```python
from build123d import *

# Parameters (mm, degrees)
F1_DEPTH = 1.5875


# Not quite as in the source:
# - a length typed as a fraction of an inch, garbled in the dataset ("3 / 203.2 mm" for 3/8 in), is restored


with BuildPart() as f1:
    # F0 (on Front) → F1 (new body)
    with BuildSketch(Plane.XZ):
        with BuildLine():
            ThreePointArc((-0.162727133, 0.4717287226), (0.0926759109, 0.1300044324), (0.4990071217, 0))
            Line((0.4990071217, 0), (22.65, 0))
            ThreePointArc((22.65, 0), (23.1449747468, 0.2050252532), (23.35, 0.7))
            Line((23.35, 0.7), (23.35, 7.5980762114))
            Line((23.35, 7.5980762114), (23.35, 8))
            Line((23.35, 8), (-12.65, 17.6461709275))
            Line((-12.65, 17.6461709275), (-12.65, 16.1461709275))
            ThreePointArc((-12.65, 16.1461709275), (-12.2964466094, 15.9997243181), (-12.15, 15.6461709275))
            ThreePointArc((-12.15, 15.6461709275), (-12.2964466094, 15.2926175369), (-12.65, 15.1461709275))
            Line((-12.65, 15.1461709275), (-12.65, 7.6820693124))
            Line((-12.65, 7.6820693124), (-6.2143365838, 7.6820693124))
            ThreePointArc((-6.2143365838, 7.6820693124), (-3.311970792, 6.7534662239), (-1.4876633356, 4.3125784367))
            Line((-1.4876633356, 4.3125784367), (-0.162727133, 0.4717287226))
        make_face()
        with BuildLine():
            Line((-13.95, 7.6820693124), (-12.65, 7.6820693124))
            Line((-12.65, 7.6820693124), (-12.65, 15.1461709275))
            ThreePointArc((-12.65, 15.1461709275), (-13.15, 15.6461709275), (-12.65, 16.1461709275))
            Line((-12.65, 16.1461709275), (-12.65, 17.6461709275))
            Line((-12.65, 17.6461709275), (-13.7688266684, 17.9459596298))
            ThreePointArc((-13.7688266684, 17.9459596298), (-14.3761330003, 17.8251588896), (-14.65, 17.2698115514))
            Line((-14.65, 17.2698115514), (-14.65, 8.3820693124))
            ThreePointArc((-14.65, 8.3820693124), (-14.4449747468, 7.8870945656), (-13.95, 7.6820693124))
        make_face()
        Polygon((23.35, 8), (23.35, 7.5980762114), (24.85, 7.5980762114), align=None)
    extrude(amount=F1_DEPTH)


solid = f1.part
```
Model file for the job. Use its own axes, mm. A direction names the side the tool comes from. Coordinates: 2 decimals unless noted, no trailing zeros. Loops run counter-clockwise (first coordinate to the right, second up) from the corner with the lowest first, then second, coordinate; pieces in that order, holes last. Notation, with made-up numbers: M -32.75,18.25 L -12.75,18.25 A18 ccw -12.75,50.25 Z; hole C 16,12.25 d11. An arc over 180 degrees is marked long. Use CSV: the item, a comma, the result in double quotes. Start each with the question number.
1. Flat gauge pins, fed straight in: pin 1 (0.8 mm diameter, centred on y = -0.5, z = 4, fed in from +X); pin 2 (0.8 mm diameter, centred on x = 24, y = -0.5, fed in from -Z). Where does each tip first touch, or does it go through?
2. Band-saw the part on B-B, the plane x = 8. List the corners of the cut face in (y, z), then the cut area to 3 significant figures.
3. Band-saw the part on C-C, the plane z = 10. List the corners of the cut face in (x, y).
4. Band-saw the part on A-A, the plane y = -0.6. List the corners of the cut face in (x, z), then the cut area to 3 significant figures.
5. Probe probe 1 along X at (y, z) = (-0.6, 1.5); probe 2 along X at (y, z) = (-0.6, 6.5); probe 3 along Z at (x, y) = (5, -1.4). List the from-to ranges inside material, lowest first. Write a range as [from, to].
6. Tool access for faces 1 (the flat face through (-10, -1, 7.682)), 2 (the flat face through (-14.65, -1, 13)), 3 (the flat face through (23.35, -1, 4)): list every direction of +Z, -Z, +X, -X, +Y, -Y with a clear straight run to the whole face (end or side of a thin tool).
Entries:
1,pin 1,"stops at x = 23.35"
1,pin 2,"stops at z = 7.6"
2,outline,"M -1.59,0 L 0,0 L 0,12.11 L -1.59,12.11 Z"
2,area,"19.2 mm2"
3,outline,"M -14.65,-1.59 L 15.89,-1.59 L 15.89,0 L -14.65,0 Z"
4,outline,"M -14.65,8.38 A0.7 ccw -13.95,7.68 L -6.21,7.68 A5 cw -1.49,4.31 L -0.16,0.47 A0.7 ccw 0.5,0 L 22.65,0 A0.7 ccw 23.35,0.7 L 23.35,7.6 L 24.85,7.6 L -13.77,17.95 A0.7 ccw -14.65,17.27 Z; hole C -12.65,15.65 d1"
4,area,"397 mm2"
5,probe 1,"x = [-0.52, 23.35]"
5,probe 2,"x = [-2.99, 23.35]"
5,probe 3,"z = [0, 12.92]"
6,face 1,"-Z, -X, +Y, -Y"
6,face 2,"+Z, -Z, -X, +Y, -Y"
6,face 3,"-Z, +X, +Y, -Y"
